Autodesk Inventor part; units mm, degrees
ref_plane "Work Plane1" through (0, -6.5, -1) normal (-1, 0, 0) x (0, 0, 1)
ref_plane "YZ Plane" through (0, 0, 0) normal (1, 0, 0) x (0, 1, 0)
ref_plane "XZ Plane" through (0, 0, 0) normal (0, 1, 0) x (-1, 0, 0)
sketch "Sketch1" plane through (0, 0, 0) normal (0, 1, 0) x (-1, 0, 0)
  line L0 (-5, 16.5) -> (-5, -1)
  line L1 (-5, -1) -> (-6, -1)
  line L2 (-6, -1) -> (-6, -16.5)
  line L3 (-6, -16.5) -> (-7, -16.5)
  line L4 (-7, -16.5) -> (-7, 1)
  line L5 (-7, 1) -> (-6, 1)
  line L6 (-6, 1) -> (-6, 16.5)
  line L7 (-6, 16.5) -> (-5, 16.5)
  line L8 (0, 14.862) -> (0, -14.862)
  line L9 (-6, 1) -> (-6, -1) construction
  point P0 (0, 0)
  point P1 (0, 0)
  point P2 (-6, 0)
  dimension "d0" = 12
  dimension "d1" = 10
  dimension "d2" = 33
  dimension "d3" = 2
  dimension "d20" = 1
extrude "Extrusion1" add sketch "Sketch1" along normal mid plane 13
sketch "Sketch2" plane through (7, -6.5, -16.5) normal (1, 0, 0) x (0, 0, -1)
  arc A0 (-26.5, 13) -> (-26.5, 0) centre (-26.5, 6.5) ccw
  line L0 (-17.5, 13) -> (-17.5, 0)
  line L1 (-33, 13) -> (-17.5, 13)
  line L2 (-33, 13) -> (-33, 0)
  line L3 (-17.5, 0) -> (-33, 0)
  line L4 (0, 13) -> (0, 0)
  line L5 (-17.5, 13) -> (0, 13)
  line L6 (-17.5, 13) -> (-17.5, 0)
  line L7 (0, 0) -> (-17.5, 0)
  arc A1 (-6.5, 0) -> (-6.5, 13) centre (-6.5, 6.5) ccw
  circle A2 centre (-6.5, 6.5) radius 2.5
  circle A3 centre (-26.5, 6.5) radius 2.5
  line L8 (-15.5, 13) -> (-33, 13)
  line L9 (-26.5, 13) -> (-33, 13)
  line L10 (-33, 13) -> (-33, 0)
  line L11 (0, 0) -> (-17.5, 0)
  line L12 (-6.5, 0) -> (0, 0)
  line L13 (0, 0) -> (0, 13)
  line L14 (-17.5, 13) -> (0, 13)
  line L15 (-6.5, 13) -> (0, 13)
  point P0 (-16.5, 6.5)
  dimension "d6" = 5
  dimension "d7" = 5
extrude "Extrusion2" cut sketch "Sketch2" against normal through all contours A0 L2 L1 | A0 L3 L2 | A1 L4 L7 | L5 L4 A1 | A2
extrude "Extrusion3" add sketch "Sketch2" along normal blind 0.5 and the other way blind 1.5 contours A3
ref_plane "Work Plane1" through (0, -6.5, -1) normal (-1, 0, 0) x (0, 0, 1)
mirror "Mirror1" about plane through (0, -6.5, -1) normal (-1, 0, 0)
sketch "Sketch3" plane through (6, -6.5, -1) normal (-1, 0, 0) x (0, 0, 1)
  line L0 (2, 13) -> (-9, 13)
  line L1 (-5, 13) -> (8, 13)
  line L2 (8, 13) -> (8, 11.75)
  line L3 (8, 11.75) -> (-5, 11.75)
  line L4 (-5, 11.75) -> (-5, 13)
  circle A0 centre (-9, 6.5) radius 2.5
  circle A1 centre (11, 6.5) radius 2.5
  line L5 (-9, 0) -> (2, 0)
  line L6 (-5, 0) -> (8, 0)
  line L7 (8, 0) -> (8, 1.25)
  line L8 (8, 1.25) -> (-5, 1.25)
  line L9 (-5, 1.25) -> (-5, 0)
  point P0 (1, 6.5)
  dimension "d15" = 4
  dimension "d16" = 10.5
  dimension "d17" = 3
extrude "Extrusion4" add sketch "Sketch3" along normal up to surface (12 mm away) contours L1 L2 L3 L4 L0 | L9 L8 L7 L6 L5
fillet "Fillet1" radius 0.2 2 edges at (7.5, 0, 12.5) (-7.5, 0, 12.5)
properties part number "Esteira-fesma-S10" material "Nylon 6/6"
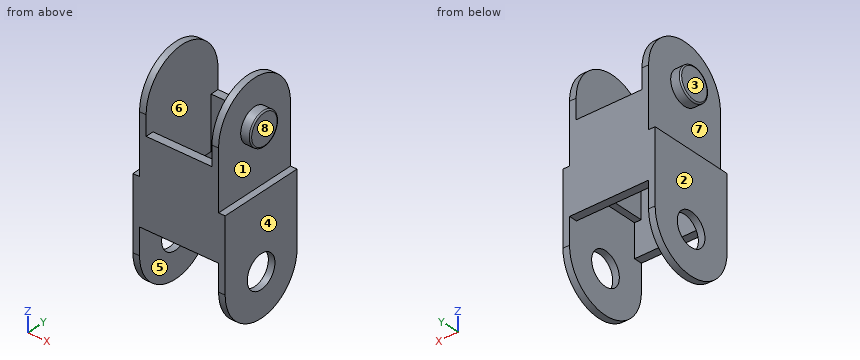
Design review of the part built by this model. Coordinates are the model's own, in mm. Face numbers are marked on the shaded views. A direction names the side the tool comes from. Round coordinates to 2 decimals unless told otherwise and drop trailing zeros. Write each loop counter-clockwise with the first axis right and the second up, starting at its lowest first coordinate (ties: lowest second). Pieces come first, ordered by that corner, then holes. Notation, with made-up numbers: (38.25, 85.25) -> (46.25, 85.25) arc R15 ccw to (46.25, 90.25) -> close; hole circle Ø1 at (32, 71). An arc over 180 degrees is marked (long way). One line per item, written item: value. Start each with the question number.
Q1. Tool access review of the marked faces 1, 2, 3, 4 and 5: name each direction out of +Z, -Z, +X, -X, +Y, -Y from which nothing blocks a thin tool from reaching the whole face with its end or side.
Q2. Add section D-D (y = 4.25). Give the boundary of the cut face in (x, z), then the cut area to 3 significant figures.
Q3. To check wall thickness, follow probe 1 along X at (y, z) = (3.25, 3); probe 2 along X at (y, z) = (-1.25, 0); probe 3 along Y at (x, z) = (-0.75, 4.5). State the ranges of each line that lie inside material, in increasing order.
Q4. Add section C-C (x = 0.5). Give the boundary of the cut face in (y, z).
Q5. Add section A-A (z = -8.5). Give the boundary of the cut face in (x, y), then the cut area to 3 significant figures.
Q6. Insertion check: P1, Ø4, axis at y = 0, z = -10, coming from the +X side; P2, Ø2, axis at x = -4.5, y = 2, coming from the -Z side; P3, Ø4, axis at x = 4.5, y = 2.5, coming from the +Z side; P4, Ø6.5, axis at y = 0, z = -10, coming from the +X side. Each pin has a flat end and moves straight along its axis. Give the tip position at first contact, or say it passes through.
Q7. Add section B-B (z = -1.5). Give the boundary of the cut face in (x, y).
Q8. The part is to be moulded in two halves that separate along X. For the marked faces 6, 7 and 8, say which applies: pulls with the +X half, pulls with the -X half, needs draft (parallel to the pull), parting line crosses it, or undercut.
Response:
1. face 1: +X
1. face 2: -Z, -X, +Y, -Y
1. face 3: +Z, -Z, -X, +Y, -Y
1. face 4: -Z, +X, +Y, -Y
1. face 5: -Z
2. outline: (-7, -14.92) -> (-6, -14.92) -> (-6, -1) -> (-5, -1) -> (-5, 14.92) -> (-6, 14.92) -> (-6, 1) -> (-7, 1) -> close; (5, -1) -> (6, -1) -> (6, -14.92) -> (7, -14.92) -> (7, 1) -> (6, 1) -> (6, 14.92) -> (5, 14.92) -> close
2. area: 63.7 mm^2
3. probe 1: x = -6 to -5, 5 to 6
3. probe 2: x = -7 to -5, 5 to 7
3. probe 3: y = -6.5 to -5.25, 5.25 to 6.5
4. outline: (-6.5, -6) -> (-5.25, -6) -> (-5.25, 7) -> (-6.5, 7) -> close; (5.25, -6) -> (6.5, -6) -> (6.5, 7) -> (5.25, 7) -> close
5. outline: (-7, -6.5) -> (-6, -6.5) -> (-6, -2) -> (-7, -2) -> close; (-7, 2) -> (-6, 2) -> (-6, 6.5) -> (-7, 6.5) -> close; (6, -6.5) -> (7, -6.5) -> (7, -2) -> (6, -2) -> close; (6, 2) -> (7, 2) -> (7, 6.5) -> (6, 6.5) -> close
5. area: 18.0 mm^2
6. P1: passes through
6. P2: stops at z = -1
6. P3: stops at z = 16.48
6. P4: stops at x = 7
7. outline: (-7, -6.5) -> (7, -6.5) -> (7, 6.5) -> (-7, 6.5) -> close; hole (-6, -5.25) -> (6, -5.25) -> (6, 5.25) -> (-6, 5.25) -> close
8. face 6: undercut
8. face 7: pulls with the -X half
8. face 8: pulls with the +X half
